Geometry: final body of the model. Coordinates: model frame, mm. A direction names the side the tool comes from. Give positions to 0.01 mm unless a question says otherwise; leave off trailing zeros. Loops run counter-clockwise (first coordinate to the right, second up) from the corner with the lowest first, then second, coordinate; pieces in that order, holes last.
1. Access query for faces 1 (the face through (8, 47, 15.875)), 2 (the face through (21.21, 72.98, 0.72)), 3 (the face through (38.1, 95.12, 8.1)), 4 (the face through (21.898, 22, 8)), 5 (the face through (34, 47.6, 7.5)). Directions: +Z, -Z, +X, -X, +Y, -Y. A direction counts if a zero-diameter tool reaches every point of the face in a straight line with its end or side. Return the directions, or none.
2. Draft query along X for faces 6 (the face through (37.76, 82.74, 7.79)), 7 (the face through (-6.057, 30.804, 9.125)), 8 (the face through (-10, 47, 4.762)). Return one class per face: +X half, -X half, draft (parallel to the pull), parting line (faces both ways), or undercut.
3. First-contact query: P1, Ø0.6, axis at y = 42.5, z = 0.5, coming from the -X side; P2, Ø5, axis at x = -6.35, y = 9.525, coming from the -Z side; P3, Ø6, axis at x = -6.35, y = 28.575, coming from the +Z side. Flat tips, straight axial feed; report the tip coordinate or a pass-through.
4. Section C-C, the plane z = 8.5. State how many separate pieces and enclosed holes the cut face has, then the cut area to 3 significant figures.
5. Material intervals for line 1 along Y through (x, z) = (-6.35, 11); line 2 along Y through (x, z) = (26.5, 14.25); line 3 along Y through (x, z) = (33, 1.25), sorted ascending.
6. Section A-A, the plane y = 76.5. Output: boundary loops of the cut face in (x, z) (1 decimal).
7. Section B-B, the plane y = 59.5. Output: boundary loops of the cut face in (x, z) (1 decimal).
from build123d import *

# Parameters (mm, degrees)
BOSS_EXTRUDE1_DEPTH                            = 95.25
CSK_FOR_8_FLAT_HEAD_MACHINE_SCREW1_D           = 4.4958
CSK_FOR_8_FLAT_HEAD_MACHINE_SCREW1_CSINK_D     = 8.4328
CSK_FOR_8_FLAT_HEAD_MACHINE_SCREW1_CSINK_ANGLE = 82
SKETCH2_R                                      = 2.9464
CUT_EXTRUDE1_DEPTH                             = 105.057346731
MOVE_FACE1_BY                                  = 0.250000008
SKETCH6_W                                      = 15.875
SKETCH6_H                                      = 19.05
CUT_EXTRUDE2_DEPTH                             = 105.057346731
MOVE_FACE2_BY                                  = 0.399999962
MOVE_FACE2_2_BY                                = 0.399999962
MOVE_FACE3_BY                                  = 1.000000032
MOVE_FACE3_2_BY                                = 1.000000032
MOVE_FACE4_BY                                  = 0.100000054
FILLET1_R                                      = 1.199999886
FILLET2_R                                      = 2.400000026
CHAMFER1_SIZE                                  = 0.799999924
CHAMFER2_SIZE                                  = 1.199999886
CUT_EXTRUDE3_DEPTH                             = 0.799999924


with BuildPart() as part:
    # Sketch1 → Boss-Extrude1 (new body)
    with BuildSketch(Plane(origin=(0, 0, 0), x_dir=(1, 0, 0), z_dir=(0, 1, 0))):
        with BuildLine():
            Line((-15.875, -4.7625), (-15.875, -15.875))
            Line((-15.875, -15.875), (30.8356, -15.875))
            ThreePointArc((30.8356, -15.875), (38.7731, -7.9375), (30.8356, 0))
            Line((30.8356, 0), (0, 0))
            Line((0, 0), (0, -4.7625))
            Line((0, -4.7625), (-15.875, -4.7625))
        make_face()
    extrude(amount=BOSS_EXTRUDE1_DEPTH)

    # CSK for #8 Flat Head Machine Screw1 (through all)
    with Locations(Plane.XY.offset(15.875)):
        with Locations((-6.35, 85.725), (-6.35, 66.675), (-6.35, 47.625), (-6.35, 28.575), (-6.35, 9.525)):
            CounterSinkHole(CSK_FOR_8_FLAT_HEAD_MACHINE_SCREW1_D / 2, CSK_FOR_8_FLAT_HEAD_MACHINE_SCREW1_CSINK_D / 2, counter_sink_angle=CSK_FOR_8_FLAT_HEAD_MACHINE_SCREW1_CSINK_ANGLE)

    # Sketch2 → Cut-Extrude1 (cut, through all)
    with BuildSketch(Plane(origin=(0, 95.25, 0), x_dir=(1, 0, 0), z_dir=(0, 1, 0))):
        with Locations(Location((30.8356, -7.9375, 0), (0, 0, 270))):
            Circle(SKETCH2_R)
    extrude(amount=-CUT_EXTRUDE1_DEPTH, mode=Mode.SUBTRACT)

    # Move Face1: a curved face moved inward by 0.25
    add(Solid.thicken(part.faces().sort_by_distance((30.8356, 47.625, 4.9911))[0], -MOVE_FACE1_BY), mode=Mode.SUBTRACT)

    # Sketch6 → Cut-Extrude2 (cut, through all)
    with BuildSketch(Plane.XY.offset(15.875)):
        with Locations((30.8356, 73.025)):
            Rectangle(SKETCH6_W, SKETCH6_H)
        with Locations((30.8356, 22.225)):
            Rectangle(SKETCH6_W, SKETCH6_H)
    extrude(amount=-CUT_EXTRUDE2_DEPTH, mode=Mode.SUBTRACT)

    # Move Face2: a face moved inward by 0.4
    extrude(part.faces().sort_by_distance((30.8356, 12.7, 3.96875))[0], amount=MOVE_FACE2_BY, dir=(0, -1, 0), mode=Mode.SUBTRACT)

    # Move Face2 2: a face moved inward by 0.4
    extrude(part.faces().sort_by_distance((30.8356, 63.5, 3.96875))[0], amount=MOVE_FACE2_2_BY, dir=(0, -1, 0), mode=Mode.SUBTRACT)

    # Move Face3: a face moved inward by 1.0
    extrude(part.faces().sort_by_distance((22.8981, 72.825000019, 7.9375))[0], amount=MOVE_FACE3_BY, dir=(-1, 0, 0), mode=Mode.SUBTRACT)

    # Move Face3 2: a face moved inward by 1.0
    extrude(part.faces().sort_by_distance((22.8981, 22.025000019, 7.9375))[0], amount=MOVE_FACE3_2_BY, dir=(-1, 0, 0), mode=Mode.SUBTRACT)

    # Move Face4: a curved face moved outward by 0.1
    add(Solid.thicken(part.faces().sort_by_distance((30.8356, 6.150000019, 4.741099992))[0], MOVE_FACE4_BY))

    # Fillet1
    fillet1_edges = [part.edges().sort_by_distance(p)[0] for p in [
        (-15.875, 47.625, 15.875),
    ]]
    fillet(fillet1_edges, radius=FILLET1_R)

    # Fillet2
    fillet2_edges = [part.edges().sort_by_distance(p)[0] for p in [
        (21.898099968, 72.825000019, 0),
        (21.898099968, 72.825000019, 15.875),
        (21.898099968, 22.025000019, 0),
        (21.898099968, 22.025000019, 15.875),
    ]]
    fillet(fillet2_edges, radius=FILLET2_R)

    # Chamfer1
    chamfer1_edges = [part.edges().sort_by_distance(p)[0] for p in [
        (8.080299943, 95.25, 15.875),
        (8.080299943, 0, 15.875),
        (-15.523528171, 0, 15.523528171),
        (-15.523528171, 95.25, 15.523528171),
        (38.7731, 95.25, 7.9375),
        (15.4178, 95.25, 0),
        (15.4178, 0, 0),
        (38.7731, 0, 7.9375),
        (-15.875, 0, 9.718750057),
        (-15.875, 95.25, 9.718750057),
    ]]
    chamfer(chamfer1_edges, length=CHAMFER1_SIZE)

    # Chamfer2
    chamfer2_edges = [part.edges().sort_by_distance(p)[0] for p in [
        (38.7731, 82.55, 7.9375),
        (25.166849971, 82.55, 0),
        (25.166849971, 63.100000038, 0),
        (38.7731, 63.100000038, 7.9375),
        (25.166849971, 82.55, 15.875),
        (25.166849971, 63.100000038, 15.875),
        (38.7731, 31.75, 7.9375),
        (25.166849971, 31.75, 0),
        (25.166849971, 12.300000038, 0),
        (38.7731, 12.300000038, 7.9375),
        (25.166849971, 31.75, 15.875),
        (25.166849971, 12.300000038, 15.875),
    ]]
    chamfer(chamfer2_edges, length=CHAMFER2_SIZE)


with BuildPart() as body_2:
    # Mirror1: mirrored copy
    add(part.part.mirror(Plane(origin=(0, 0, 0), x_dir=(0, 0, 1), z_dir=(1, 0, 0))))


with BuildPart() as cut_extrude3_tool:
    # Sketch7 → Cut-Extrude3 (new body)
    # profile 1 of 2: a face of its own
    with BuildSketch(Plane(origin=(0, 0, 0), x_dir=(-1, 0, 0), z_dir=(0, 0, -1))):
        with BuildLine():
            Line((-20.412409211, 38.1), (-21.734237952, 38.1))
            Line((-21.734237952, 38.1), (-23.320432442, 40.743657484))
            add(Edge.make_bspline(
                [(-23.320432442, 40.743657484), (-23.39246628, 40.858422627), (-23.52796777, 41.074305166), (-23.74573892, 41.362084605), (-23.956458509, 41.605820363), (-24.178959725, 41.796609957), (-24.411259949, 41.945774465), (-24.66555501, 42.041863685), (-24.94306761, 42.100661436), (-25.137376333, 42.107127078), (-25.239531949, 42.110526316)],
                knots=[0, 0, 0, 0, 1.306497362, 2.457627467, 3.478958043, 4.407874435, 5.276294006, 6.127627337, 7.015621229, 8, 8, 8, 8], degree=3))
            Line((-25.239531949, 42.110526316), (-26.177540789, 42.110526316))
            Line((-26.177540789, 42.110526316), (-26.177540789, 38.1))
            Line((-26.177540789, 38.1), (-27.305501316, 38.1))
            Line((-27.305501316, 38.1), (-27.305501316, 47.625))
            Line((-27.305501316, 47.625), (-24.450351234, 47.625))
            add(Edge.make_bspline(
                [(-24.450351234, 47.625), (-24.347806001, 47.623129418), (-24.146199259, 47.619451803), (-23.849497415, 47.590158509), (-23.565748079, 47.538652332), (-23.294428494, 47.470652115), (-23.037326038, 47.383677735), (-22.797710845, 47.273159326), (-22.57435286, 47.144015465), (-22.370417771, 46.991886303), (-22.183160925, 46.822598362), (-22.019334584, 46.629590128), (-21.876320998, 46.418408005), (-21.756058405, 46.187155813), (-21.659502559, 45.936474231), (-21.588740249, 45.664775603), (-21.547846501, 45.371631063), (-21.542908146, 45.169465091), (-21.540369737, 45.065547903)],
                knots=[0, 0, 0, 0, 1.122660118, 2.207180616, 3.260035189, 4.277559223, 5.267526261, 6.226939943, 7.162224589, 8.087074141, 9.00774428, 9.920166118, 10.85183919, 11.794874382, 12.767769948, 13.787074559, 14.862513871, 16, 16, 16, 16], degree=3))
            add(Edge.make_bspline(
                [(-21.540369737, 45.065547903), (-21.542357217, 44.983878967), (-21.546264084, 44.823339156), (-21.57390063, 44.587383869), (-21.620526513, 44.361103987), (-21.687741358, 44.145993266), (-21.769898701, 43.941469561), (-21.868344577, 43.74780219), (-21.984139869, 43.565845661), (-22.115072733, 43.395259432), (-22.261958201, 43.238149058), (-22.419872875, 43.089916318), (-22.595585255, 42.957356067), (-22.784024282, 42.835490164), (-22.985181681, 42.726560713), (-23.198195231, 42.629572918), (-23.423773409, 42.547595818), (-23.579934628, 42.503184465), (-23.659212253, 42.480638363)],
                knots=[0, 0, 0, 0, 1.081472828, 2.125893282, 3.141472299, 4.136796786, 5.106410527, 6.057503338, 7.009617098, 7.958900923, 8.9009934, 9.855302418, 10.823566394, 11.811505165, 12.825021642, 13.850268175, 14.908655843, 16, 16, 16, 16], degree=3))
            Line((-23.659212253, 42.480638363), (-23.659212253, 42.453222656))
            add(Edge.make_bspline(
                [(-23.659212253, 42.453222656), (-23.580440976, 42.417398664), (-23.430201665, 42.349072086), (-23.227647339, 42.216467885), (-23.043792737, 42.06881687), (-22.876744064, 41.892393409), (-22.707999377, 41.696943007), (-22.5465086, 41.468307362), (-22.37186832, 41.212866322), (-22.253430103, 41.030490431), (-22.190513651, 40.933609169)],
                knots=[0, 0, 0, 0, 0.964360555, 1.839310864, 2.693732611, 3.590073818, 4.546144586, 5.573387662, 6.710941094, 8, 8, 8, 8], degree=3))
            Line((-22.190513651, 40.933609169), (-20.412409211, 38.1))
        make_face()
        with BuildLine():
            Line((-26.177540789, 46.622368421), (-26.177540789, 43.113157895))
            Line((-26.177540789, 43.113157895), (-24.638344655, 43.113157895))
            add(Edge.make_bspline(
                [(-24.638344655, 43.113157895), (-24.569102811, 43.114710218), (-24.432171893, 43.117780052), (-24.230682013, 43.140672174), (-24.038064572, 43.183371896), (-23.852785081, 43.236317079), (-23.679677481, 43.310303445), (-23.515001668, 43.393491968), (-23.365110484, 43.494164986), (-23.225565012, 43.605761469), (-23.10263029, 43.734919697), (-22.990088563, 43.874377459), (-22.896446885, 44.030414223), (-22.812645632, 44.196203849), (-22.749245008, 44.376780257), (-22.701600246, 44.56741074), (-22.674241595, 44.768408501), (-22.670326553, 44.905542676), (-22.668330263, 44.975467722)],
                knots=[0, 0, 0, 0, 1.090010243, 2.155576699, 3.185466336, 4.1933334, 5.183762916, 6.144316812, 7.093369302, 8.020984545, 8.951157476, 9.894798401, 10.83591824, 11.810170468, 12.814521676, 13.841330878, 14.899289422, 16, 16, 16, 16], degree=3))
            add(Edge.make_bspline(
                [(-22.668330263, 44.975467722), (-22.669755188, 45.038210828), (-22.672541335, 45.160892047), (-22.696634379, 45.339904799), (-22.73515642, 45.508714327), (-22.790191358, 45.666401453), (-22.860981229, 45.813536083), (-22.950346987, 45.948264178), (-23.05196724, 46.074873626), (-23.170530652, 46.18917611), (-23.304284867, 46.289915007), (-23.449590319, 46.382158658), (-23.611610469, 46.455601424), (-23.787524875, 46.51610884), (-23.976521707, 46.565569479), (-24.180601911, 46.597218806), (-24.397597512, 46.620398699), (-24.547543149, 46.62169958), (-24.624636801, 46.622368421)],
                knots=[0, 0, 0, 0, 1.036630811, 2.02691802, 2.979521427, 3.89397019, 4.781810153, 5.670567375, 6.560240909, 7.460578941, 8.384147086, 9.324204361, 10.29927051, 11.31606129, 12.396781476, 13.52306989, 14.726501219, 16, 16, 16, 16], degree=3))
            Line((-24.624636801, 46.622368421), (-26.177540789, 46.622368421))
        make_face(mode=Mode.SUBTRACT)
    # profile 2 of 2: a face of its own
    with BuildSketch(Plane(origin=(0, 0, 0), x_dir=(-1, 0, 0), z_dir=(0, 0, -1))):
        Polygon((27.430830263, 38.1), (22.543001316, 38.1), (22.543001316, 47.625), (23.670961842, 47.625), (23.670961842, 39.102631579), (27.430830263, 39.102631579), align=None)
    extrude(amount=-CUT_EXTRUDE3_DEPTH)


with BuildPart() as part_1:
    add(part.part)

    # Cut-Extrude3: cut by cut_extrude3_tool
    add(cut_extrude3_tool.part, mode=Mode.SUBTRACT)


with BuildPart() as body_2_1:
    add(body_2.part)

    # Cut-Extrude3: cut by cut_extrude3_tool
    add(cut_extrude3_tool.part, mode=Mode.SUBTRACT)


solid = part_1.part
Answers below:
1. face 1: +Z, +X, -X, +Y, -Y
1. face 2: -Z, +X
1. face 3: +X, +Y
1. face 4: +Z, -Z, +X
1. face 5: +Y
2. face 6: +X half
2. face 7: undercut
2. face 8: draft
3. P1: stops at x = 0
3. P2: stops at z = 4.76
3. P3: stops at z = 14.48
4. separate pieces: 4
4. enclosed holes: 5
4. area: 4,110 mm2
5. line 1: y = 0 to 7.28, 11.77 to 26.33, 30.82 to 45.38, 49.87 to 64.43, 68.92 to 83.48, 87.97 to 95.25
5. line 2: y = 0 to 12.3, 31.75 to 63.1, 82.55 to 95.25
5. line 3: y = 0 to 12.01, 32.04 to 62.81, 82.84 to 95.25
6. outline: (-15.9, 4.8) - (0, 4.8) - (0, 0) - (19.5, 0) arc R2.4 ccw to (21.9, 2.4) - (21.9, 13.5) arc R2.4 ccw to (19.5, 15.9) - (-14.7, 15.9) arc R1.2 ccw to (-15.9, 14.7) - close
7. outline: (-15.9, 4.8) - (0, 4.8) - (0, 0) - (30.8, 0) arc R7.9 ccw to (30.8, 15.9) - (-14.7, 15.9) arc R1.2 ccw to (-15.9, 14.7) - close; hole circle Ø6.4 at (30.8, 7.9)
